Job drawing, mm, ordinate dimensions from the low corner. One solid piece. Round coordinates to 2 decimals unless told otherwise and drop trailing zeros. Order: outer loops, then holes, each group sorted by start corner. A loop starts at its lowest first (then second) coordinate and runs counter-clockwise, first axis right, second up. Notation, with made-up numbers: (47, 34) -> (90, 34) arc R17 cw to (90, 43) -> close; hole circle Ø6 at (1, 15). An arc over 180 degrees is marked (long way). Use CSV: the item, a comma, the result in double quotes.
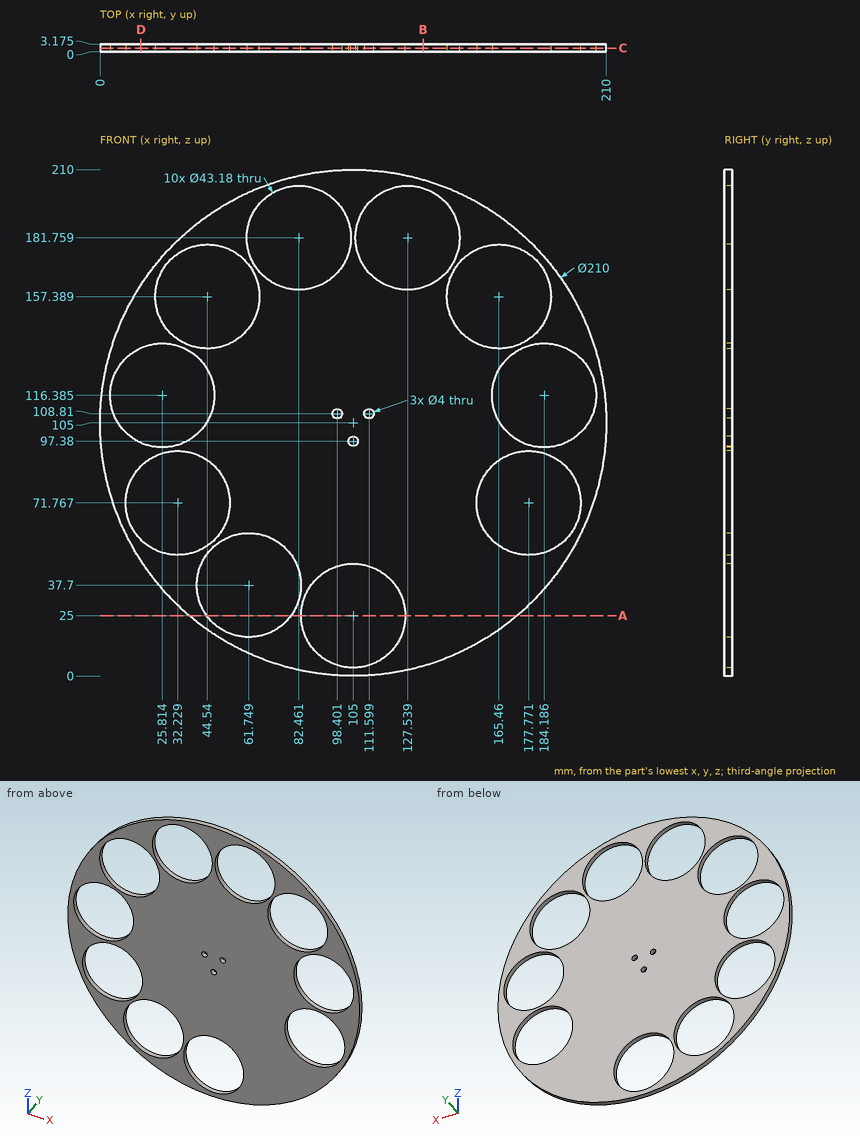
(1) Probe probe 1 along X at (y, z) = (0.8, 106.5); probe 2 along X at (y, z) = (1.7, 78); probe 3 along X at (y, z) = (1.6, 108.81). List the from-to ranges inside material, lowest first. Write a range as [from, to].
Reply:
probe 1,"[0.01, 6.62], [45.01, 164.99], [203.38, 209.99]"
probe 2,"[3.53, 11.56], [52.9, 157.1], [198.44, 206.47]"
probe 3,"[0.07, 5.6], [46.03, 96.4], [100.4, 109.6], [113.6, 163.97], [204.4, 209.93]"
(2) Cut at C-C, the plane y = 1.5. State how many separate pieces and enclosed holes the cut face has, then the cut area to 3 significant figures.
Reply:
separate pieces,"1"
enclosed holes,"13"
area,"20,000 mm2"
(3) Cut at A-A, the plane z = 25. Give the cut face in (x, y) (1 decimal), then the cut area to 3 significant figures.
Reply:
outline,"(37, 0) -> (44.3, 0) -> (44.3, 3.2) -> (37, 3.2) -> close; (79.2, 0) -> (83.4, 0) -> (83.4, 3.2) -> (79.2, 3.2) -> close; (126.6, 0) -> (173, 0) -> (173, 3.2) -> (126.6, 3.2) -> close"
area,"184 mm2"
(4) Cut at D-D, the plane x = 17. Give the cut face in (y, z) (1 decimal), then the cut area to 3 significant figures.
Reply:
outline,"(0, 47.7) -> (3.2, 47.7) -> (3.2, 56.5) -> (0, 56.5) -> close; (0, 87.1) -> (3.2, 87.1) -> (3.2, 96.7) -> (0, 96.7) -> close; (0, 136.1) -> (3.2, 136.1) -> (3.2, 162.3) -> (0, 162.3) -> close"
area,"141 mm2"
(5) Cut at B-B, the plane x = 134. Give the cut face in (y, z) (1 decimal), then the cut area to 3 significant figures.
Reply:
outline,"(0, 4.1) -> (3.2, 4.1) -> (3.2, 161.2) -> (0, 161.2) -> close; (0, 202.4) -> (3.2, 202.4) -> (3.2, 205.9) -> (0, 205.9) -> close"
area,"510 mm2"
